Geometry check sheet. Reference: the model listing, model coordinates, mm. Face numbers are marked on the shaded views. A direction names the side the tool comes from. Round coordinates to 2 decimals unless told otherwise and drop trailing zeros. Write each loop counter-clockwise with the first axis right and the second up, starting at its lowest first coordinate (ties: lowest second). Pieces come first, ordered by that corner, then holes. Notation, with made-up numbers: M -21.75,-21.75 L 25.25,-21.75 A14 ccw 25.25,-6.75 Z; hole C 46,-29.5 d2. An arc over 180 degrees is marked long. Use a Markdown table: item, result.
Autodesk Inventor part; units mm, degrees
ref_plane "YZ Plane" through (0, 0, 0) normal (1, 0, 0) x (0, 1, 0)
ref_plane "XZ Plane" through (0, 0, 0) normal (0, 1, 0) x (-1, 0, 0)
ref_plane "XY Plane" through (0, 0, 0) normal (0, 0, 1) x (1, 0, 0)
sketch "Sketch1" plane through (0, 0, 0) normal (1, 0, 0) x (0, 1, 0)
  line L0 (0, 0) -> (65, 0)
  line L1 (65, 0) -> (65, 48)
  line L2 (65, 48) -> (0, 48)
  line L3 (0, 48) -> (0, 0)
  dimension "d0" = 65
  dimension "d1" = 48
extrude "Extrusion1" add sketch "Sketch1" against normal blind 40
sketch "Sketch2" plane through (0, 0, 0) normal (1, 0, 0) x (0, 0, -1)
  line L0 (-36.5, 45) -> (-11.5, 45) construction
  line L1 (-11.5, 45) -> (-11.5, 20) construction
  line L2 (-11.5, 20) -> (-36.5, 20) construction
  line L3 (-36.5, 20) -> (-36.5, 45) construction
  line L4 (-36.5, 45) -> (-36.5, 65) construction
  line L5 (-48, 65) -> (0, 65) construction
  line L6 (-36.5, 45) -> (-48, 45) construction
  line L7 (-48, 0) -> (-48, 65) construction
  line L8 (-11.5, 20) -> (-11.5, 0) construction
  line L9 (0, 0) -> (-48, 0) construction
  line L10 (-11.5, 20) -> (0, 20) construction
  circle A0 centre (-36.5, 45) radius 2
  circle A1 centre (-11.5, 45) radius 2
  circle A2 centre (-11.5, 20) radius 2
  circle A3 centre (-36.5, 20) radius 2
  line L11 (0, 0) -> (0, 65)
  dimension "d4" = 25
  dimension "d5" = 25
  dimension "d6" = 4
  dimension "d7" = 4
  dimension "d8" = 4
  dimension "d9" = 4
extrude "Extrusion2" cut sketch "Sketch2" against normal blind 8
sketch "Sketch3" plane through (0, 0, 48) normal (0, 0, 1) x (1, 0, 0)
  line L0 (0, 65) -> (0, 0) construction
  line L1 (0, 32.5) -> (-40, 32.5) construction
  line L2 (-40, 0) -> (-40, 65) construction
  line L3 (-25, 32.5) -> (-15, 32.5) construction
  circle A0 centre (-25, 32.5) radius 1.5
  circle A1 centre (-15, 32.5) radius 1.5
  dimension "d12" = 10
  dimension "d13" = 15
  dimension "d14" = 3
  dimension "d15" = 3
extrude "Extrusion3" cut sketch "Sketch3" against normal blind 6
sketch "Sketch4" plane through (0, 0, 0) normal (0, 0, -1) x (-1, 0, 0)
  circle A0 centre (25, 32.5) radius 1.5
  circle A1 centre (15, 32.5) radius 1.5
  point P0 (0, 0)
extrude "Extrusion4" cut sketch "Sketch4" against normal blind 6
thread "Thread1"
thread "Thread2"
thread "Thread3"
thread "Thread4"
thread "Thread5"
thread "Thread6"
thread "Thread7"
thread "Thread8"
sketch "Sketch5" plane through (0, 65, 48) normal (0, 1, 0) x (1, 0, 0)
  line L0 (-40, 48) -> (-40, 0)
  line L1 (-40, 10.5) -> (-40, 37.5)
  line L2 (0, 0) -> (0, 48)
  line L3 (0, 10.5) -> (0, 37.5)
  line L4 (0, 38.5) -> (-8, 38.5)
  arc A0 (-40, 10.5) -> (0, 10.5) centre (-20, 24.2976) ccw
  arc A1 (0, 37.5) -> (-40, 37.5) centre (-20, 23.7024) ccw
  line L5 (-0.01, 10.5031) -> (-0.01, 37.4969)
  arc A2 (-0.01, 37.4969) -> (-39.99, 37.4969) centre (-20, 23.7024) ccw
  line L6 (-39.99, 37.4969) -> (-39.99, 10.5031)
  arc A3 (-39.99, 10.5031) -> (-0.01, 10.5031) centre (-20, 24.2976) ccw
  line L7 (-39.99, 24) -> (-0.01, 24) construction
  circle A4 centre (-20, 24) radius 8
  dimension "d36" = 27
  dimension "d37" = 10.5
  dimension "d38" = 0.01
  dimension "d39" = 16
extrude "Extrusion5" add sketch "Sketch5" along normal blind 10 contours A2 L5 A3 L6
sketch "Sketch6" plane through (0, 75, 48) normal (0, 1, 0) x (1, 0, 0)
  arc A0 (-0.01, 37.4969) -> (-39.99, 37.4969) centre (-20, 23.7024) ccw
  line L0 (-39.99, 37.4969) -> (-39.99, 10.5031)
  arc A1 (-39.99, 10.5031) -> (-0.01, 10.5031) centre (-20, 24.2976) ccw
  line L1 (-0.01, 10.5031) -> (-0.01, 37.4969)
  circle A2 centre (-20, 24) radius 8
  arc A3 (-5.01, 35.8396) -> (-34.99, 35.8396) centre (-20, 23.7024) ccw construction
  line L2 (-5.01, 35.8396) -> (-5.01, 12.1604) construction
  arc A4 (-34.99, 12.1604) -> (-5.01, 12.1604) centre (-20, 24.2976) ccw construction
  line L3 (-34.99, 12.1604) -> (-34.99, 35.8396) construction
  circle A5 centre (-34.99, 35.8396) radius 4.25
  circle A6 centre (-20, 42.99) radius 4.25
  circle A7 centre (-5.01, 35.8396) radius 4.25
  circle A8 centre (-5.01, 12.1604) radius 4.25
  circle A9 centre (-20, 5.01) radius 4.25
  circle A10 centre (-34.99, 12.1604) radius 4.25
  point P0 (0, 48)
  dimension "d42" = 5
  dimension "d43" = 8.5
  dimension "d44" = 8.5
  dimension "d45" = 8.5
  dimension "d46" = 8.5
  dimension "d47" = 8.5
  dimension "d48" = 8.5
extrude "Extrusion6" add sketch "Sketch6" along normal blind 4.75 contours A5 | A6 | A7 | A8 | A9 | A10
sketch "Sketch7" plane through (-20, 65, 24) normal (0, 1, 0) x (1, 0, 0)
  circle A0 centre (0, 0) radius 8
  point P0 (20, 24)
extrude "Extrusion7" cut sketch "Sketch7" against normal up to next
equation "\"d7\" = d6"
equation "\"d8\" = d6"
equation "\"d9\" = d6"
equation "\"d15\" = d14"
equation "\"d44\" = d43"
equation "\"d45\" = d43"
equation "\"d46\" = d43"
equation "\"d47\" = d43"
equation "\"d48\" = d43"
properties part number "Z Axis Statonary Block"
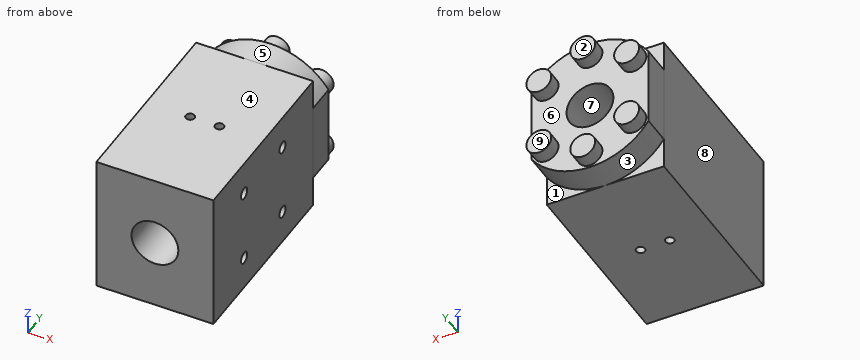
Item 1: Cross-section at D-D, the plane x = -5.01. Record the cut outline in (y, z), and give its area (3 significant figures).
Outcome:
| item | result |
|---|---|
| outline | M 0,0 L 65,0 L 65,5.19 L 75,5.19 L 75,7.91 L 79.75,7.91 L 79.75,16.41 L 75,16.41 L 75,31.59 L 79.75,31.59 L 79.75,40.09 L 75,40.09 L 75,42.81 L 65,42.81 L 65,48 L 0,48 Z; hole C 20,11.5 d4; hole C 20,36.5 d4; hole C 45,11.5 d4; hole C 45,36.5 d4 |
| area | 3,530 mm2 |
Item 2: Go/stop test with flat-tipped pins: pin 1 (3.5 mm diameter, centred on x = -15, y = 32.5, fed in from +Z); pin 2 (1.2 mm diameter, centred on y = 45, z = 35.5, fed in from +X); pin 3 (8 mm diameter, centred on y = 71, z = 25, fed in from -X); pin 4 (1.8 mm diameter, centred on x = -15, y = 32.5, fed in from +Z). Record where each tip stops, or that it passes through.
Outcome:
| item | result |
|---|---|
| pin 1 | stops at z = 48 |
| pin 2 | stops at x = -8 |
| pin 3 | stops at x = -39.99 |
| pin 4 | stops at z = 42 |
Item 3: Material ranges on line 1 along Y through (x, z) = (-4.5, 11.5); line 2 along Y through (x, z) = (-2, 11); line 3 along X through (y, z) = (32, 4), recorded low to high. Write a range as from..to.
Outcome:
| item | result |
|---|---|
| line 1 | y = 0..18, 22..43, 47..79.75 |
| line 2 | y = 0..18.06, 21.94..43.06, 46.94..79.75 |
| line 3 | x = -40..-26.41, -23.59..-16.41, -13.59..0 |
Item 4: Access from +Z, -Z, +X, -X, +Y, -Y to the whole of each face (thin tool, end or side, straight path). Record for the marked faces 1, 2, 3, 4 and 5.
Outcome:
| item | result |
|---|---|
| face 1 | +Y |
| face 2 | +Z, -Z, +X, -X, +Y |
| face 3 | -Z, +Y |
| face 4 | +Z, +X, -X, +Y, -Y |
| face 5 | +Z, +Y |
Item 5: Mould release check, pull along X, two halves, no side actions. Record for the marked faces 6, 7, 8 and 9: +X half, -X half, draft (parallel to the pull), parting line (faces both ways), or undercut.
Outcome:
| item | result |
|---|---|
| face 6 | undercut |
| face 7 | undercut |
| face 8 | -X half |
| face 9 | draft |
Item 6: Cross-section at C-C, the plane y = 20. Record the cut outline in (x, z).
Outcome:
| item | result |
|---|---|
| outline | M -40,0 L 0,0 L 0,9.5 L -8,9.5 L -8,13.5 L 0,13.5 L 0,34.5 L -8,34.5 L -8,38.5 L 0,38.5 L 0,48 L -40,48 Z; hole C -20,24 d16 |
